Geometry: final body of the model. Coordinates: model frame, mm. A direction names the side the tool comes from. Give positions to 0.01 mm unless a question says otherwise; leave off trailing zeros. Write each loop counter-clockwise with the first axis right and the second up, starting at its lowest first coordinate (ties: lowest second). Pieces come first, ordered by that corner, then holes. Notation, with made-up numbers: (28, 64.5) -> (42, 64.5) arc R22 cw to (42, 98.5) -> close; hole circle Ø9 at (-24, -6.75). An arc over 180 degrees is marked (long way). Answer as a JSON object with one key per item and string values.
from build123d import *

# Parameters (mm, degrees)
SKETCH1_R           = 2.5
SKETCH1_R_2         = 2
BASE_FLANGE1_DEPTH  = 3
EDGE_FLANGE1_DEPTH  = 16
SKETCH10_R          = 2.5
CUT_EXTRUDE1_DEPTH  = 10
TAB1_START          = -3
TAB1_DEPTH          = 3
SWEEP1_PROFILE_R    = 2
BOSS_EXTRUDE1_START = 15
SKETCH35_R          = 2
BOSS_EXTRUDE1_DEPTH = 15


# Read off the part's stored shape, not the designer's step: Tab1
# Sheet-metal steps are written as plain solids
with BuildPart() as part:
    # Sketch1 → Base-Flange1 (new body)
    with BuildSketch(Plane(origin=(0, 0, 0), x_dir=(1, 0, 0), z_dir=(0, 1, 0))):
        with BuildLine():
            Line((0, -8), (-7, -8))
            ThreePointArc((-7, -8), (-15, 0), (-7, 8))
            Line((-7, 8), (0, 8))
            Line((0, 8), (15, 8))
            Line((15, 8), (15, -8))
            Line((15, -8), (0, -8))
        make_face()
        with Locations(Location((0, 0, 0), (0, 0, 270))):
            Circle(SKETCH1_R, mode=Mode.SUBTRACT)
        with Locations(Location((-7, 0, 0), (0, 0, 270))):
            Circle(SKETCH1_R_2, mode=Mode.SUBTRACT)
    extrude(amount=-BASE_FLANGE1_DEPTH)

    # Edge-Flange1 section (across the edge) → Edge-Flange1 (add)
    with BuildSketch(Plane(origin=(15.7366, 0, 8), x_dir=(-1, 0, 0), z_dir=(0, 0, -1))):
        with BuildLine():
            Line((-3, 0.7366), (-3, 17))
            Line((-3, 17), (0, 17))
            Line((0, 17), (0, 0.7366))
            ThreePointArc((0, 0.7366), (0.215745145, 0.215745145), (0.7366, 0))
            Line((0.7366, 0), (0.7366, -3))
            ThreePointArc((0.7366, -3), (-1.905575199, -1.905575199), (-3, 0.7366))
        make_face()
    extrude(amount=EDGE_FLANGE1_DEPTH)

    # Sketch10 → Cut-Extrude1 (cut)
    with BuildSketch(Plane.ZY.offset(-15.7366)):
        with BuildLine():
            Line((-8, 17), (-8, 9))
            ThreePointArc((-8, 9), (-5.656854249, 14.656854249), (0, 17))
            Line((0, 17), (-8, 17))
        make_face()
        with BuildLine():
            Line((8, 17), (0, 17))
            ThreePointArc((0, 17), (5.656854249, 14.656854249), (8, 9))
            Line((8, 9), (8, 17))
        make_face()
        with Locations(Location((0, 9, 0), (0, 0, 270))):
            Circle(SKETCH10_R)
    extrude(amount=-CUT_EXTRUDE1_DEPTH, mode=Mode.SUBTRACT)


with BuildPart() as body_2:
    # Mirror1: mirrored copy
    add(part.part.mirror(Plane.XY.offset(-19)))


with BuildPart() as part_1:
    add(part.part)

    add(body_2.part)  # Tab1 merges body 2
    # Tab1 outline → Tab1 (add)
    with BuildSketch(Plane.ZY.offset(-15.7366).offset(TAB1_START)):
        with BuildLine():
            ThreePointArc((-8, 9), (-5.656854249, 14.656854249), (0, 17))
            Line((0, 17), (-38, 17))
            ThreePointArc((-38, 17), (-32.343145751, 14.656854249), (-30, 9))
            Line((-30, 9), (-30, 0.7366))
            Line((-30, 0.7366), (-8, 0.7366))
            Line((-8, 0.7366), (-8, 9))
        make_face()
    extrude(amount=TAB1_DEPTH)



with BuildPart() as body_2_2:
    # Sweep1: sweep along a path in Sketch15
    with BuildLine(Plane.ZY.offset(7)) as sweep1_path:
        ThreePointArc((0, -3), (-19, -22), (-38, -3))
    # Sweep1 profile (on start of the path) → Sweep1 (sweep)
    with BuildSketch(Plane(origin=(-7, -3, 0), x_dir=(-1, 0, 0), z_dir=(0, -1, 0))):
        Circle(SWEEP1_PROFILE_R)
    sweep(path=sweep1_path.line)


with BuildPart() as part_2:
    add(part_1.part)

    add(body_2_2.part)  # Boss-Extrude1 merges body 2 2
    # Sketch35 → Boss-Extrude1 (add)
    with BuildSketch(Plane(origin=(0, -3, 0), x_dir=(1, 0, 0), z_dir=(0, 1, 0)).offset(BOSS_EXTRUDE1_START)):
        with Locations(Location((-7, 38, 0), (0, 0, 90))):
            Circle(SKETCH35_R)
        with Locations(Location((-7, 0, 0), (0, 0, 270))):
            Circle(SKETCH35_R)
    extrude(amount=-BOSS_EXTRUDE1_DEPTH)


solid = part_2.part
Q1. Material intervals for L1, parallel to X at y = 13, z = -1.5; L2, parallel to X at y = -1, z = 0; L3, parallel to Z at x = -2, y = -1, sorted ascending. Write a range as from..to.
Values:
{"L1": "15.74..18.74", "L2": "-15..-2.5, 2.5..18.31", "L3": "-46..-39.5, -36.5..-30, -8..-1.5, 1.5..8"}
Q2. Cut plane A-A (x = 12). Return the cut outline in (y, z).
Values:
{"outline": "(-3, -46) -> (0, -46) -> (0, -30) -> (-3, -30) -> close; (-3, -8) -> (0, -8) -> (0, 8) -> (-3, 8) -> close"}
Q3. Set-up query: faces 1 (the cylindrical face through (-7, 6, -36)), 2 (the flat face through (17, 17, -19)), 3 (the cylindrical face through (17.2, 11.5, 0.1)). Return all of +Z, -Z, +X, -X, +Y, -Y with unobstructed straight access to the full face (end or side cutting, diameter ignored); none if empty.
Values:
{"face 1": "+Y", "face 2": "+Z, -Z, +X, -X, +Y", "face 3": "+X"}
Q4. Cut plane C-C (x = 0). Return the cut outline in (y, z), and give its area (3 significant figures).
Values:
{"outline": "(-3, -46) -> (0, -46) -> (0, -40.5) -> (-3, -40.5) -> close; (-3, -35.5) -> (0, -35.5) -> (0, -30) -> (-3, -30) -> close; (-3, -8) -> (0, -8) -> (0, -2.5) -> (-3, -2.5) -> close; (-3, 2.5) -> (0, 2.5) -> (0, 8) -> (-3, 8) -> close", "area": "66.0 mm²"}
Q5. First-contact query: P1, Ø5, axis at y = -10.5, z = -5.5, coming from the -X side; P2, Ø0.9, axis at x = 17.5, z = -20.5, coming from the -Y side; P3, Ø8, axis at x = -2.5, z = -26.5, coming from the -Y side; P4, Ø3, axis at x = 0, z = 0, coming from the -Y side. Flat tips, straight axial feed; report the tip coordinate or a pass-through.
Values:
{"P1": "x = -8.7", "P2": "y = 0.74", "P3": "y = -22.97", "P4": "through"}
Q6. Cut plane B-B (y = 3.5). Return the cut outline in (x, z), and give its area (3 significant figures).
Values:
{"outline": "circle Ø4 at (-7, -38); circle Ø4 at (-7, 0); (15.74, -46) -> (18.74, -46) -> (18.74, 8) -> (15.74, 8) -> close", "area": "187 mm²"}
Q7. Mould query, pull axis X, two halves, no side actions, for faces 4 (the cylindrical face through (17.613, -1.934, 0.112)), 5 (the flat face through (-7, 12, -38)), 6 (the flat face through (4, 0, 0)), 7 (the cylindrical face through (-7, 6, -2)). Classes: pulls with the +X half, pulls with the -X half, needs draft (parallel to the pull), parting line crosses it, or undercut.
Values:
{"face 4": "pulls with the +X half", "face 5": "needs draft", "face 6": "undercut", "face 7": "undercut"}
